Input: part model. Units: mm. Frame: model coordinates. Give positions to 0.01 mm unless a question says otherwise; leave off trailing zeros. Loops run counter-clockwise (first coordinate to the right, second up) from the corner with the lowest first, then second, coordinate; pieces in that order, holes last. Notation, with made-up numbers: (-12, 88) - (18, 88) arc R15 cw to (18, 92) - close; hole circle Ø2 at (15, 19.25). An arc over 180 degrees is marked (long way). One line per question, with ' | ' between items. Start each with the question number.
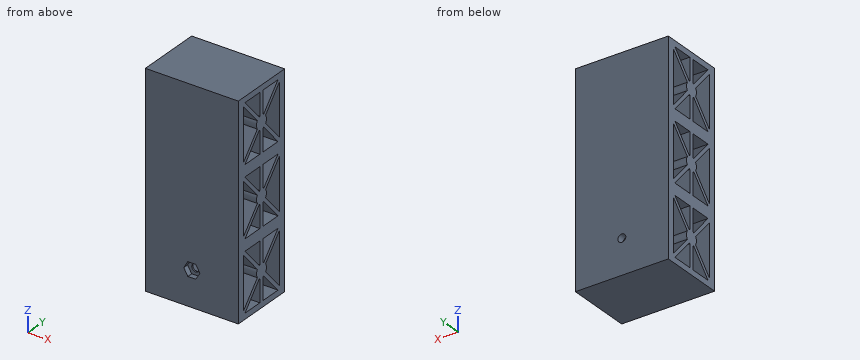
from build123d import *

# Parameters (mm, degrees)
SKETCH19_W          = 30
SKETCH19_H          = 28
SKETCH19_W_2        = 25
SKETCH19_H_2        = 22
BOSS_EXTRUDE1_DEPTH = 40
BOSS_EXTRUDE2_DEPTH = 40
LPATTERN2_COUNT     = 3
LPATTERN2_PITCH     = 30
SKETCH22_R          = 1.7
CUT_EXTRUDE1_DEPTH  = 29
CUT_EXTRUDE2_DEPTH  = 2.32


with BuildPart() as part:
    # Sketch19 → Boss-Extrude1 (new body)
    with BuildSketch(Plane(origin=(0, 0, 0), x_dir=(0, 0, -1), z_dir=(1, 0, 0))):
        with Locations((1, -10)):
            Rectangle(SKETCH19_W, SKETCH19_H)
        with Locations((1, -10)):
            Rectangle(SKETCH19_W_2, SKETCH19_H_2, mode=Mode.SUBTRACT)
    extrude(amount=-BOSS_EXTRUDE1_DEPTH)

    # Sketch21 → Boss-Extrude2 (add)
    with BuildSketch(Plane(origin=(0, 0, 0), x_dir=(0, 0, -1), z_dir=(1, 0, 0))):
        with BuildLine():
            Line((-11.995470921, 0.436964862), (-1.676096633, -8.644084511))
            ThreePointArc((-1.676096633, -8.644084511), (-1.252140551, -8.018116315), (-0.68515479, -7.518014236))
            Line((-0.68515479, -7.518014236), (-11.004529079, 1.563035138))
            Line((-11.004529079, 1.563035138), (-11.995470921, 0.436964862))
        make_face()
        with BuildLine():
            Line((13.004529079, 1.563035138), (2.68515479, -7.518014236))
            ThreePointArc((2.68515479, -7.518014236), (3.252140551, -8.018116315), (3.676096633, -8.644084511))
            Line((3.676096633, -8.644084511), (13.995470921, 0.436964862))
            Line((13.995470921, 0.436964862), (13.004529079, 1.563035138))
        make_face()
        with BuildLine():
            Line((-1.828427125, -9), (-11.5, -9))
            Line((-11.5, -9), (-11.5, -11))
            Line((-11.5, -11), (-1.828427125, -11))
            ThreePointArc((-1.828427125, -11), (-2, -10), (-1.828427125, -9))
        make_face()
        with BuildLine():
            Line((13.5, -9), (3.828427125, -9))
            ThreePointArc((3.828427125, -9), (3.956795679, -9.492694064), (4, -10))
            ThreePointArc((4, -10), (3.956795679, -10.507305936), (3.828427125, -11))
            Line((3.828427125, -11), (13.5, -11))
            Line((13.5, -11), (13.5, -9))
        make_face()
        with BuildLine():
            ThreePointArc((-0.68515479, -12.481985764), (-1.252140551, -11.981883685), (-1.676096633, -11.355915489))
            Line((-1.676096633, -11.355915489), (-11.995470921, -20.436964862))
            Line((-11.995470921, -20.436964862), (-11.004529079, -21.563035138))
            Line((-11.004529079, -21.563035138), (-0.68515479, -12.481985764))
        make_face()
        with BuildLine():
            ThreePointArc((3.676096633, -11.355915489), (3.252140551, -11.981883685), (2.68515479, -12.481985764))
            Line((2.68515479, -12.481985764), (13.004529079, -21.563035138))
            Line((13.004529079, -21.563035138), (13.995470921, -20.436964862))
            Line((13.995470921, -20.436964862), (3.676096633, -11.355915489))
        make_face()
        with BuildLine():
            Line((-1.271647214, -9), (-1.828427125, -9))
            ThreePointArc((-1.828427125, -9), (-2, -10), (-1.828427125, -11))
            Line((-1.828427125, -11), (-1.271647214, -11))
            Line((-1.271647214, -11), (-0.135283578, -10))
            Line((-0.135283578, -10), (-1.271647214, -9))
        make_face()
        with BuildLine():
            Line((3.828427125, -9), (3.271647214, -9))
            Line((3.271647214, -9), (2.135283578, -10))
            Line((2.135283578, -10), (3.271647214, -11))
            Line((3.271647214, -11), (3.828427125, -11))
            ThreePointArc((3.828427125, -11), (3.956795679, -10.507305936), (4, -10))
            ThreePointArc((4, -10), (3.956795679, -9.492694064), (3.828427125, -9))
        make_face()
        with BuildLine():
            ThreePointArc((-1.676096633, -8.644084511), (-1.758009138, -8.81958245), (-1.828427125, -9))
            Line((-1.828427125, -9), (-1.271647214, -9))
            Line((-1.271647214, -9), (-1.676096633, -8.644084511))
        make_face()
        with BuildLine():
            Line((-1.676096633, -8.644084511), (-1.271647214, -9))
            Line((-1.271647214, -9), (0.998919941, -9))
            Line((0.998919941, -9), (-0.68515479, -7.518014236))
            ThreePointArc((-0.68515479, -7.518014236), (-1.252140551, -8.018116315), (-1.676096633, -8.644084511))
        make_face()
        Polygon((0.998919941, -9), (-1.271647214, -9), (-0.135283578, -10), (1, -9.000950452), align=None)
        with BuildLine():
            Line((-1.271647214, -11), (-1.828427125, -11))
            ThreePointArc((-1.828427125, -11), (-1.758009138, -11.18041755), (-1.676096633, -11.355915489))
            Line((-1.676096633, -11.355915489), (-1.271647214, -11))
        make_face()
        with BuildLine():
            Line((-0.68515479, -7.518014236), (0.998919941, -9))
            Line((0.998919941, -9), (1.001080059, -9))
            Line((1.001080059, -9), (2.68515479, -7.518014236))
            ThreePointArc((2.68515479, -7.518014236), (1, -7), (-0.68515479, -7.518014236))
        make_face()
        Polygon((1.001080059, -9), (0.998919941, -9), (1, -9.000950452), align=None)
        Polygon((1, -10.999049548), (-0.135283578, -10), (-1.271647214, -11), (0.998919941, -11), align=None)
        Polygon((1, -9.000950452), (-0.135283578, -10), (1, -10.999049548), (2.135283578, -10), align=None)
        with BuildLine():
            Line((0.998919941, -11), (-1.271647214, -11))
            Line((-1.271647214, -11), (-1.676096633, -11.355915489))
            ThreePointArc((-1.676096633, -11.355915489), (-1.252140551, -11.981883685), (-0.68515479, -12.481985764))
            Line((-0.68515479, -12.481985764), (0.998919941, -11))
        make_face()
        with BuildLine():
            Line((2.68515479, -7.518014236), (1.001080059, -9))
            Line((1.001080059, -9), (3.271647214, -9))
            Line((3.271647214, -9), (3.676096633, -8.644084511))
            ThreePointArc((3.676096633, -8.644084511), (3.252140551, -8.018116315), (2.68515479, -7.518014236))
        make_face()
        Polygon((3.271647214, -9), (1.001080059, -9), (1, -9.000950452), (2.135283578, -10), align=None)
        Polygon((1.001080059, -11), (1, -10.999049548), (0.998919941, -11), align=None)
        Polygon((2.135283578, -10), (1, -10.999049548), (1.001080059, -11), (3.271647214, -11), align=None)
        with BuildLine():
            Line((1.001080059, -11), (0.998919941, -11))
            Line((0.998919941, -11), (-0.68515479, -12.481985764))
            ThreePointArc((-0.68515479, -12.481985764), (1, -13), (2.68515479, -12.481985764))
            Line((2.68515479, -12.481985764), (1.001080059, -11))
        make_face()
        with BuildLine():
            Line((3.676096633, -8.644084511), (3.271647214, -9))
            Line((3.271647214, -9), (3.828427125, -9))
            ThreePointArc((3.828427125, -9), (3.758009138, -8.81958245), (3.676096633, -8.644084511))
        make_face()
        with BuildLine():
            Line((3.271647214, -11), (1.001080059, -11))
            Line((1.001080059, -11), (2.68515479, -12.481985764))
            ThreePointArc((2.68515479, -12.481985764), (3.252140551, -11.981883685), (3.676096633, -11.355915489))
            Line((3.676096633, -11.355915489), (3.271647214, -11))
        make_face()
        with BuildLine():
            Line((3.828427125, -11), (3.271647214, -11))
            Line((3.271647214, -11), (3.676096633, -11.355915489))
            ThreePointArc((3.676096633, -11.355915489), (3.758009138, -11.18041755), (3.828427125, -11))
        make_face()
    extrude(amount=-BOSS_EXTRUDE2_DEPTH)


with BuildPart() as lpattern2_1:
    # LPattern2: pattern copy
    add(part.part.moved(Location(Vector(0, 0, 1) * (1 * LPATTERN2_PITCH))))


with BuildPart() as lpattern2_2:
    # LPattern2: pattern copy
    add(part.part.moved(Location(Vector(0, 0, 1) * (2 * LPATTERN2_PITCH))))


with BuildPart() as part_1:
    add(part.part)

    # Sketch22 → Cut-Extrude1 (cut, through all)
    with BuildSketch(Plane(origin=(0, 4, 0), x_dir=(1, 0, 0), z_dir=(0, 1, 0))):
        with Locations((-20, 1)):
            Circle(SKETCH22_R)
    extrude(amount=-CUT_EXTRUDE1_DEPTH, mode=Mode.SUBTRACT)

    # Sketch32 → Cut-Extrude2 (cut)
    with BuildSketch(Plane(origin=(0, -24, 0), x_dir=(-1, 0, 0), z_dir=(0, -1, 0))):
        Polygon((16.535898385, 1), (18.267949192, -2), (21.732050808, -2), (23.464101615, 1), (21.732050808, 4), (18.267949192, 4), align=None)
    extrude(amount=-CUT_EXTRUDE2_DEPTH, mode=Mode.SUBTRACT)

    # Combine1: union LPattern2_1, LPattern2_2
    add(lpattern2_1.part)
    add(lpattern2_2.part)


solid = part_1.part
Q1. Line query: L1, parallel to X at y = 2.2, z = -1; L2, parallel to Y at x = -7.5, z = 58; L3, parallel to Y at x = -36, z = -0.5. Output: solid intervals per line, ascending. Write a range as from..to.
Q2. Section B-B, the plane x = -15. Count the separate pieces of the cut face and the enclosed holes in it, plus the area to 3 significant figures.
Q3. First-contact query: pin 1 (5.5 mm diameter, centred on x = -20, z = -1, fed in from -Y). Flat tip, straight axial feed; report the tip coordinate or a pass-through.
Q4. Section A-A, the plane z = -7.5. Output: boundary loops of the cut face in (x, y).
Solved:
1) L1: x = -40..-21.7, -18.3..0 | L2: y = -24..-21, -12.83..-7.17, 1..4 | L3: y = -24..-21, -12.96..-7.04, 1..4
2) separate pieces: 1 | enclosed holes: 18 | area: 1,310 mm²
3) pin 1: stops at y = -21.68
4) outline: (-40, -24) - (0, -24) - (0, -21) - (-40, -21) - close; (-40, -16.72) - (0, -16.72) - (0, -14.72) - (-40, -14.72) - close; (-40, -11) - (0, -11) - (0, -9) - (-40, -9) - close; (-40, -5.28) - (0, -5.28) - (0, -3.28) - (-40, -3.28) - close; (-40, 1) - (0, 1) - (0, 4) - (-40, 4) - close
